Design review of the part built by this model. Coordinates are the model's own, in mm. A direction names the side the tool comes from. Round coordinates to 2 decimals unless told otherwise and drop trailing zeros. Write each loop counter-clockwise with the first axis right and the second up, starting at its lowest first coordinate (ties: lowest second). Pieces come first, ordered by that corner, then holes. Notation, with made-up numbers: M 61.25,14.25 L 90.25,14.25 A31 cw 90.25,53.25 Z; hole C 72.25,11 d9. An arc over 180 degrees is marked long. Use CSV: the item, a comma, the result in double quotes.
from build123d import *

# Parameters (mm, degrees)
F0_R     = 9.525
F1_DEPTH = 76.2


with BuildPart() as f1:
    # F0 (on Top) → F1 (new body)
    with BuildSketch(Plane.XY):
        with BuildLine():
            ThreePointArc((14.261609, -6.972958), (0, -15.875), (-14.261609, -6.972958))
            Line((-14.261609, -6.972958), (-10.796512, -14.06003))
            ThreePointArc((-10.796512, -14.06003), (-10.410981, -15.146229), (-10.280226, -16.291377))
            Line((-10.280226, -16.291377), (-10.280226, -19.044231))
            ThreePointArc((-10.280226, -19.044231), (-11.768124, -22.636333), (-15.360226, -24.124231))
            Line((-15.360226, -24.124231), (-26.940812, -24.124231))
            Line((-26.940812, -24.124231), (-26.940812, -27.02905))
            Line((-26.940812, -27.02905), (26.940812, -27.02905))
            Line((26.940812, -27.02905), (26.940812, -24.124231))
            Line((26.940812, -24.124231), (15.360226, -24.124231))
            ThreePointArc((15.360226, -24.124231), (11.768124, -22.636333), (10.280226, -19.044231))
            Line((10.280226, -19.044231), (10.280226, -16.291377))
            ThreePointArc((10.280226, -16.291377), (10.410981, -15.146229), (10.796512, -14.06003))
            Line((10.796512, -14.06003), (14.261609, -6.972958))
        make_face()
        with BuildLine():
            ThreePointArc((14.261609, -6.972958), (15.466394, -3.578588), (15.875, 0))
            ThreePointArc((15.875, 0), (-3.578588, 15.466394), (-14.261609, -6.972958))
            ThreePointArc((-14.261609, -6.972958), (0, -15.875), (14.261609, -6.972958))
        make_face()
        Circle(F0_R, mode=Mode.SUBTRACT)
    extrude(amount=F1_DEPTH)


solid = f1.part
1) Add section B-B on z = 64. Write out the cut boundary in (x, y) (3 decimals).
Answers:
outline,"M -26.941,-27.029 L 26.941,-27.029 L 26.941,-24.124 L 15.36,-24.124 A5.08 cw 10.28,-19.044 L 10.28,-16.291 A5.08 cw 10.797,-14.06 L 14.262,-6.973 A15.875 ccw 15.875,0 A15.875 ccw long -14.262,-6.973 L -10.797,-14.06 A5.08 cw -10.28,-16.291 L -10.28,-19.044 A5.08 cw -15.36,-24.124 L -26.941,-24.124 Z; hole C 0,0 d19.05"
2) Machinability: for faces 4 (the face through (10.28, -18, 38)), 5 (the face through (0, -10, 0)), 6 (the face through (-12.55, -10.47, 37.57)), which of the approach directions +Z, -Z, +X, -X, +Y, -Y give a long, thin tool a straight path to every point of the face, cutting with its end or side? Answer none if there is none.
Answers:
face 4,"+Z, -Z, +X"
face 5,"-Z, +X, -X, +Y, -Y"
face 6,"+Z, -Z, -X"
3) Add section D-D on y = -18. Write out the cut boundary in (x, z).
Answers:
outline,"M -10.28,0 L 10.28,0 L 10.28,76.2 L -10.28,76.2 Z"
4) Wall thickness on line 1 along Y through (x, z) = (0, 45.5) (3 decimals); line 2 along X through (y, z) = (-3, 22.5); line 3 along Y through (x, z) = (7, 50): over which ranges is each line inside the solid? List them lowest first. Write a range as [from, to].
Answers:
line 1,"[-27.029, -9.525], [9.525, 15.875]"
line 2,"[-15.59, -9.04], [9.04, 15.59]"
line 3,"[-27.03, -6.46], [6.46, 14.25]"
5) For pin 1 Ø8 at (y, z) = (1, 41.5) entering from +X (3 decimals); pin 2 Ø6 at (x, z) = (-20.5, 39) entering from +Y; pin 3 Ø17 at (x, y) = (0, 0) entering from -Z; pin 4 Ø10 at (y, z) = (-8.5, 15) entering from -X, all flat-tipped, find the tip position at first contact; note any pin that passes through.
Answers:
pin 1,"x = 15.875"
pin 2,"y = -24.12"
pin 3,"through"
pin 4,"x = -15.48"
6) Add section A-A on x = 0. Write out the cut boundary in (y, z) (3 decimals).
Answers:
outline,"M -27.029,0 L -9.525,0 L -9.525,76.2 L -27.029,76.2 Z; M 9.525,0 L 15.875,0 L 15.875,76.2 L 9.525,76.2 Z"
7) Add section C-C on x = -6. Write out the cut boundary in (y, z), then the cut area to 3 significant figures.
Answers:
outline,"M -27.03,0 L -7.4,0 L -7.4,76.2 L -27.03,76.2 Z; M 7.4,0 L 14.7,0 L 14.7,76.2 L 7.4,76.2 Z"
area,"2,050 mm²"
8) The part is to be moulded in two halves that separate along Y. For faces 1 (the face through (11.81, -22.68, 37.57)), 2 (the face through (0, -27.029, 38)), 3 (the face through (26.941, -26, 38)), say which applies: released by +Y, released by -Y, zero draft, split by the parting line, or undercut.
Answers:
face 1,"undercut"
face 2,"released by -Y"
face 3,"zero draft"
